from build123d import *

# Parameters (mm, degrees)
CROQUIS1_W              = 200
CROQUIS1_H              = 101.6
SALIENTE_EXTRUIR1_DEPTH = 12.7
CROQUIS2_W              = 200
CROQUIS2_H              = 12.7
SALIENTE_EXTRUIR2_DEPTH = 101.6
CROQUIS3_R              = 2.783946769
CROQUIS3_R_2            = 2.839641003
CROQUIS3_R_3            = 2.758984083
CROQUIS3_R_4            = 2.686508842
CROQUIS3_R_5            = 2.837304272
CROQUIS3_R_6            = 2.927811787
CROQUIS3_R_7            = 2.625457287
CROQUIS3_R_8            = 2.715964801
CORTAR_EXTRUIR1_DEPTH   = 101.6


with BuildPart() as part:
    # Croquis1 → Saliente-Extruir1 (new body)
    with BuildSketch(Plane(origin=(0, 0, 0), x_dir=(0, 0, -1), z_dir=(1, 0, 0))):
        Rectangle(CROQUIS1_W, CROQUIS1_H)
    extrude(amount=SALIENTE_EXTRUIR1_DEPTH)

    # Croquis2 → Saliente-Extruir2 (add)
    with BuildSketch(Plane(origin=(12.7, 0, 0), x_dir=(0, 0, -1), z_dir=(1, 0, 0))):
        with Locations((0, 44.45)):
            Rectangle(CROQUIS2_W, CROQUIS2_H)
    extrude(amount=SALIENTE_EXTRUIR2_DEPTH)

    # Croquis3 → Cortar-Extruir1 (cut)
    with BuildSketch(Plane(origin=(12.7, 0, 0), x_dir=(0, 0, -1), z_dir=(1, 0, 0))):
        with Locations((-80, -3.526056283)):
            Circle(CROQUIS3_R)
        with Locations((-45, -3.526056283)):
            Circle(CROQUIS3_R_2)
        with Locations((-80, -38.526056283)):
            Circle(CROQUIS3_R_3)
        with Locations((-45, -38.526056283)):
            Circle(CROQUIS3_R_4)
        with Locations((40, 0)):
            Circle(CROQUIS3_R_5)
        with Locations((75, 0)):
            Circle(CROQUIS3_R_6)
        with Locations((40, -35)):
            Circle(CROQUIS3_R_7)
        with Locations((75, -35)):
            Circle(CROQUIS3_R_8)
    extrude(amount=-CORTAR_EXTRUIR1_DEPTH, mode=Mode.SUBTRACT)


solid = part.part
Model file for the job. Use its own axes, mm. A direction names the side the tool comes from. Give positions to 0.01 mm unless a question says otherwise; leave off trailing zeros. Order: outer loops, then holes, each group sorted by start corner. A loop starts at its lowest first (then second) coordinate and runs counter-clockwise, first axis right, second up. Notation, with made-up numbers: M -31.75,28.25 L -3.75,28.25 A20 ccw -3.75,60.25 Z; hole C -3.75,-14.75 d7. An arc over 180 degrees is marked long. Put each result on its own line as item: value. Start each with the question number.
(1) Band-saw the part on C-C on z = 45. Give the cut face in (x, y).
(2) Tool access for faces 4 (the face through (114.3, 45, 1)), 5 (the face through (12.7, -6, 1)): list every direction of +Z, -Z, +X, -X, +Y, -Y with a clear straight run to the whole face (end or side of a thin tool).
(3) Band-saw the part on D-D on y = -15.5. Give the cut face in (x, z), then the cut area to 3 significant figures.
(4) Pin check, flat tips, straight feed: pin 1 Ø9 at (y, z) = (-3.53, 80) entering from +X; pin 2 Ø8 at (x, z) = (30, -53.5) entering from -Y. Stop position of each tip, or through.
(5) Band-saw the part on B-B on z = -6. Give the cut face in (x, y).
(6) Pull direction Y, two halves, no side cores. Call faces 1 (the face through (36, 41, -100)), 2 (the face through (6.439, -3.401, 47.837)), 3 (the face through (56, 50.8, 1)): released by +Y, released by -Y, zero draft, split by the parting line, or undercut.
(7) Drill centre lines: L1, parallel to Y at x = 7, z = -75; L2, parallel to Y at x = 4, z = 80; L3, parallel to X at y = 1, z = 88. Where is each one in solid material? Low to high. Write a range as [from, to].
(8) Band-saw the part on A-A on z = -75. Give the cut face in (x, y), then the cut area to 3 significant figures.
Results below:
1. outline: M 0,-50.8 L 12.7,-50.8 L 12.7,-41.21 L 0,-41.21 Z; M 0,-35.84 L 12.7,-35.84 L 12.7,-6.37 L 0,-6.37 Z; M 0,-0.69 L 12.7,-0.69 L 12.7,38.1 L 114.3,38.1 L 114.3,50.8 L 0,50.8 Z
2. face 4: +Z, -Z, +X, +Y, -Y
2. face 5: +Z, -Z, +X, -Y
3. outline: M 0,-100 L 12.7,-100 L 12.7,100 L 0,100 Z
3. area: 2,540 mm2
4. pin 1: stops at x = 12.7
4. pin 2: stops at y = 38.1
5. outline: M 0,-50.8 L 12.7,-50.8 L 12.7,38.1 L 114.3,38.1 L 114.3,50.8 L 0,50.8 Z
6. face 1: zero draft
6. face 2: undercut
6. face 3: released by +Y
7. L1: y = [-50.8, -37.72], [-32.28, -2.93], [2.93, 50.8]
7. L2: y = [-50.8, -41.29], [-35.77, -6.31], [-0.74, 50.8]
7. L3: x = [0, 12.7]
8. outline: M 0,-50.8 L 12.7,-50.8 L 12.7,-37.72 L 0,-37.72 Z; M 0,-32.28 L 12.7,-32.28 L 12.7,-2.93 L 0,-2.93 Z; M 0,2.93 L 12.7,2.93 L 12.7,38.1 L 114.3,38.1 L 114.3,50.8 L 0,50.8 Z
8. area: 2,440 mm2
